```python
from build123d import *

# Parameters (mm, degrees)
BOX009_W               = 20
BOX009_H               = 30
BOX009_DEPTH           = 30
BOX008_W               = 70
BOX008_H               = 10
BOX008_DEPTH           = 50
BOX008_PLACEMENT_ANGLE = 90
BOX005_W               = 70
BOX005_H               = 10
BOX005_DEPTH           = 50
BOX001_W               = 10
BOX001_H               = 10
BOX001_DEPTH           = 10
BOX004_W               = 10
BOX004_H               = 10
BOX004_DEPTH           = 10
BOX003_W               = 10
BOX003_H               = 10
BOX003_DEPTH           = 10
BOX002_W               = 10
BOX002_H               = 10
BOX002_DEPTH           = 10
BOX_W                  = 30
BOX_H                  = 30
BOX_DEPTH              = 70
BOX007_W               = 70
BOX007_H               = 10
BOX007_DEPTH           = 50
BOX007_PLACEMENT_ANGLE = 90
BOX006_W               = 70
BOX006_H               = 10
BOX006_DEPTH           = 50


with BuildPart() as main_door:
    # Box009 → Box009 (new body)
    with BuildSketch(Plane(origin=(52, 0, 0), x_dir=(1, 0, 0), z_dir=(0, 0, 1))):
        with Locations((10, 15)):
            Rectangle(BOX009_W, BOX009_H)
    extrude(amount=BOX009_DEPTH)


with BuildPart() as right_wall:
    # Box008 → Box008 (new body)
    with BuildSketch(Plane.XY):
        with Locations((35, 5)):
            Rectangle(BOX008_W, BOX008_H)
    extrude(amount=BOX008_DEPTH)


with BuildPart() as right_wall_1:
    # Box008 placement: moved
    add(right_wall.part.moved(Location((120, 30, 0))).rotate(Axis((120, 30, 0), (0, 0, 1)), BOX008_PLACEMENT_ANGLE))


with BuildPart() as front_wall:
    # Box005 → Box005 (new body)
    with BuildSketch(Plane(origin=(30, 10, 0), x_dir=(1, 0, 0), z_dir=(0, 0, 1))):
        with Locations((35, 5)):
            Rectangle(BOX005_W, BOX005_H)
    extrude(amount=BOX005_DEPTH)


with BuildPart() as cube001:
    # Box001 → Box001 (new body)
    with BuildSketch(Plane.XY.offset(70)):
        with Locations((5, 5)):
            Rectangle(BOX001_W, BOX001_H)
    extrude(amount=BOX001_DEPTH)


with BuildPart() as cube004:
    # Box004 → Box004 (new body)
    with BuildSketch(Plane(origin=(20, 20, 70), x_dir=(1, 0, 0), z_dir=(0, 0, 1))):
        with Locations((5, 5)):
            Rectangle(BOX004_W, BOX004_H)
    extrude(amount=BOX004_DEPTH)


with BuildPart() as cube003:
    # Box003 → Box003 (new body)
    with BuildSketch(Plane(origin=(0, 20, 70), x_dir=(1, 0, 0), z_dir=(0, 0, 1))):
        with Locations((5, 5)):
            Rectangle(BOX003_W, BOX003_H)
    extrude(amount=BOX003_DEPTH)


with BuildPart() as cube002:
    # Box002 → Box002 (new body)
    with BuildSketch(Plane(origin=(20, 0, 70), x_dir=(1, 0, 0), z_dir=(0, 0, 1))):
        with Locations((5, 5)):
            Rectangle(BOX002_W, BOX002_H)
    extrude(amount=BOX002_DEPTH)


with BuildPart() as cube:
    # Box → Box (new body)
    with BuildSketch(Plane.XY):
        with Locations((15, 15)):
            Rectangle(BOX_W, BOX_H)
    extrude(amount=BOX_DEPTH)


with BuildPart() as fusion002:
    # Fusion002 base: copy of Cube
    add(cube.part)

    # Fusion002: union Cube001, Cube004, Cube003, Cube002
    add(cube001.part)
    add(cube004.part)
    add(cube003.part)
    add(cube002.part)


with BuildPart() as fusion002_1:
    # Fusion002 placement: moved
    add(fusion002.part.moved(Location((0, 100, 0))))


with BuildPart() as left_wall:
    # Box007 → Box007 (new body)
    with BuildSketch(Plane.XY):
        with Locations((35, 5)):
            Rectangle(BOX007_W, BOX007_H)
    extrude(amount=BOX007_DEPTH)


with BuildPart() as left_wall_1:
    # Box007 placement: moved
    add(left_wall.part.moved(Location((21, 30, 0))).rotate(Axis((21, 30, 0), (0, 0, 1)), BOX007_PLACEMENT_ANGLE))


with BuildPart() as fusion001:
    # Fusion001 base: copy of Cube
    add(cube.part)

    # Fusion001: union Cube001, Cube004, Cube003, Cube002
    add(cube001.part)
    add(cube004.part)
    add(cube003.part)
    add(cube002.part)


with BuildPart() as fusion001_1:
    # Fusion001 placement: moved
    add(fusion001.part.moved(Location((100, 0, 0))))


with BuildPart() as back_wall:
    # Box006 → Box006 (new body)
    with BuildSketch(Plane(origin=(30, 112, 0), x_dir=(1, 0, 0), z_dir=(0, 0, 1))):
        with Locations((35, 5)):
            Rectangle(BOX006_W, BOX006_H)
    extrude(amount=BOX006_DEPTH)


with BuildPart() as fusion003:
    # Fusion003 base: copy of Cube
    add(cube.part)

    # Fusion003: union Cube001, Cube004, Cube003, Cube002
    add(cube001.part)
    add(cube004.part)
    add(cube003.part)
    add(cube002.part)


with BuildPart() as fusion003_1:
    # Fusion003 placement: moved
    add(fusion003.part.moved(Location((100, 100, 0))))


with BuildPart() as castle:
    # Fusion base: copy of Cube
    add(cube.part)

    # Fusion: union Cube001, Cube004, Cube003, Cube002
    add(cube001.part)
    add(cube004.part)
    add(cube003.part)
    add(cube002.part)

    # Fusion004: union right-wall, front-wall, Fusion002, left-wall, Fusion001, back-wall, Fusion003
    add(right_wall_1.part)
    add(front_wall.part)
    add(fusion002_1.part)
    add(left_wall_1.part)
    add(fusion001_1.part)
    add(back_wall.part)
    add(fusion003_1.part)

    # Cut: cut main_door
    add(main_door.part, mode=Mode.SUBTRACT)


solid = castle.part
```
Work out the finished part from the listing and answer in its coordinate system (mm). A direction names the side the tool comes from. Round coordinates to 2 decimals unless told otherwise and drop trailing zeros. Loops run counter-clockwise (first coordinate to the right, second up) from the corner with the lowest first, then second, coordinate; pieces in that order, holes last. Notation, with made-up numbers: (62.25, -28) -> (68.25, -28) arc R9 ccw to (68.25, -24) -> close; hole circle Ø7 at (17, -20). An arc over 180 degrees is marked (long way). Write each question's results on one line, items separated by ' | '. Start each with the question number.
1. Section C-C (x = 48) is taken. Determine the outline of the cut face in (y, z).
2. For a pull along X with two mould halves and no side action, classify faces 5 (the face through (105, 5, 80)), 6 (the face through (8, 100, 39)), 7 (the face through (130, 115, 39)) as +X half, -X half, draft (parallel to the pull), parting line (faces both ways), or undercut.
3. Section A-A (y = 59.5) is taken. Determine the outline of the cut face in (x, z).
4. Section D-D (z = 58) is taken. Determine the outline of the cut face in (x, y), plus the area to 3 significant figures.
5. Given pin 1 Ø8 at (x, y) = (55, 105.5) entering from -Z; pin 2 Ø25 at (y, z) = (76, 22.5) entering from +X; pin 3 Ø12 at (x, z) = (87, 26.5) entering from -Y; pin 4 Ø11 at (x, y) = (16.5, 78) entering from +Z, each flat-ended and moving along its own axis, determine where each tip first touches the part or whether it passes through.
6. Find the intervals of material crossed by probe 1 along Y at (x, z) = (28, 72); probe 2 along X at (y, z) = (97, 33.5); probe 3 along Y at (x, z) = (25.5, 67.5), in increasing order. Write a range as from..to.
7. A tool of negligible diameter and unlimited length cuts with its end or side. For faces 1 (the face through (25, 10, 75)), 2 (the face through (125, 5, 80)), 3 (the face through (110, 65, 25)), 4 (the face through (110, 105, 75)), from which of +Z, -Z, +X, -X, +Y, -Y can it reach the whole face along a straight path? Write none if from no direction.
Evaluation:
1) outline: (10, 0) -> (20, 0) -> (20, 50) -> (10, 50) -> close; (112, 0) -> (122, 0) -> (122, 50) -> (112, 50) -> close
2) face 5: draft | face 6: undercut | face 7: +X half
3) outline: (11, 0) -> (21, 0) -> (21, 50) -> (11, 50) -> close; (110, 0) -> (120, 0) -> (120, 50) -> (110, 50) -> close
4) outline: (0, 0) -> (30, 0) -> (30, 30) -> (0, 30) -> close; (0, 100) -> (30, 100) -> (30, 130) -> (0, 130) -> close; (100, 0) -> (130, 0) -> (130, 30) -> (100, 30) -> close; (100, 100) -> (130, 100) -> (130, 130) -> (100, 130) -> close | area: 3,600 mm2
5) pin 1: passes through | pin 2: stops at x = 120 | pin 3: stops at y = 10 | pin 4: stops at z = 50
6) probe 1: y = 0..10, 20..30, 100..110, 120..130 | probe 2: x = 11..21, 110..120 | probe 3: y = 0..30, 100..130
7) face 1: +Z, +X, -X | face 2: +Z, +X, -X, +Y, -Y | face 3: +Z, -Z | face 4: +Z, +Y, -Y
